Build history of the part. All positions in model axes, mm. Give positions to 0.01 mm unless a question says otherwise; leave off trailing zeros. Write each loop counter-clockwise with the first axis right and the second up, starting at its lowest first coordinate (ties: lowest second). Pieces come first, ordered by that corner, then holes. Notation, with made-up numbers: (35, 48.5) -> (76, 48.5) arc R6 cw to (76, 57.5) -> close; hole circle Ø4 at (-22.5, 71.25). An arc over 180 degrees is marked (long way). Put each result on its own line as item: value.
from build123d import *

# Parameters (mm, degrees)
F0_W     = 39
F0_H     = 8
F0_R     = 3
F1_DEPTH = 7
F2_R     = 3.99999


# Not quite as in the source:
# - a fillet or chamfer is up to 0.001 mm smaller than in the source, because OpenCascade refuses the exact size


with BuildPart() as f1:
    # F0 (on Top) → F1 (new body)
    with BuildSketch(Plane.XY):
        Rectangle(F0_W, F0_H)
        with Locations((-16, 0)):
            Circle(F0_R, mode=Mode.SUBTRACT)
        with Locations((-8, 0)):
            Circle(F0_R, mode=Mode.SUBTRACT)
        Circle(F0_R, mode=Mode.SUBTRACT)
        with Locations((8, 0)):
            Circle(F0_R, mode=Mode.SUBTRACT)
        with Locations((16, 0)):
            Circle(F0_R, mode=Mode.SUBTRACT)
    extrude(amount=F1_DEPTH)

    # F2 (radius 4 in the source; OpenCascade refuses exactly that, so slightly less here)
    f2_edges = [f1.edges().sort_by_distance(p)[0] for p in [
        (-19.5, 4, 3.5),
        (-19.5, -4, 3.5),
        (19.5, -4, 3.5),
        (19.5, 4, 3.5),
    ]]
    fillet(f2_edges, radius=F2_R)


solid = f1.part
1) Pull direction Y, two halves, no side cores. Call faces 1 (the cylindrical face through (-18.359, -2.797, 3.549)), 2 (the cylindrical face through (-3, 0, 3)), 3 (the cylindrical face through (-18.359, 2.797, 3.549)): released by +Y, released by -Y, zero draft, split by the parting line, or undercut.
Filled sheet:
face 1: released by -Y
face 2: undercut
face 3: released by +Y
2) Slice it at B-B (y = -1.5). Write the cut outline in (x, z), plus the area to 3 significant figures.
Filled sheet:
outline: (-19.21, 0) -> (-18.6, 0) -> (-18.6, 7) -> (-19.21, 7) -> close; (-13.4, 0) -> (-10.6, 0) -> (-10.6, 7) -> (-13.4, 7) -> close; (-5.4, 0) -> (-2.6, 0) -> (-2.6, 7) -> (-5.4, 7) -> close; (2.6, 0) -> (5.4, 0) -> (5.4, 7) -> (2.6, 7) -> close; (10.6, 0) -> (13.4, 0) -> (13.4, 7) -> (10.6, 7) -> close; (18.6, 0) -> (19.21, 0) -> (19.21, 7) -> (18.6, 7) -> close
area: 87.0 mm2
3) Slice it at C-C (x = -8). Write the cut outline in (y, z), plus the area to 3 significant figures.
Filled sheet:
outline: (-4, 0) -> (-3, 0) -> (-3, 7) -> (-4, 7) -> close; (3, 0) -> (4, 0) -> (4, 7) -> (3, 7) -> close
area: 14.0 mm2
4) Slice it at D-D (x = 1). Write the cut outline in (y, z), plus the area to 3 significant figures.
Filled sheet:
outline: (-4, 0) -> (-2.83, 0) -> (-2.83, 7) -> (-4, 7) -> close; (2.83, 0) -> (4, 0) -> (4, 7) -> (2.83, 7) -> close
area: 16.4 mm2
5) Slice it at A-A (z = 2.75). Give the number of separate pieces and of enclosed holes in the cut face, plus the area to 3 significant figures.
Filled sheet:
separate pieces: 1
enclosed holes: 5
area: 157 mm2
6) Wall check: L1, parallel to Y at x = 0, z = 4; L2, parallel to X at y = 1.25, z = 6; L3, parallel to X at y = 2.75, z = 1. Give the ranges that are in metal, low to high.
Filled sheet:
L1: -4 to -3, 3 to 4
L2: -19.3 to -18.73, -13.27 to -10.73, -5.27 to -2.73, 2.73 to 5.27, 10.73 to 13.27, 18.73 to 19.3
L3: -18.4 to -17.2, -14.8 to -9.2, -6.8 to -1.2, 1.2 to 6.8, 9.2 to 14.8, 17.2 to 18.4
7) Pin check, flat tips, straight feed: pin 1 (3.5 mm diameter, centred on x = 0, y = 0, fed in from -Z); pin 2 (2 mm diameter, centred on y = 1.5, z = 1, fed in from +X). Stop position of each tip, or through.
Filled sheet:
pin 1: through
pin 2: x = 19.47
